For this review, take the finished solid that the model builds, in its own axes (mm). Face numbers are marked on the shaded views. A direction names the side the tool comes from. Round coordinates to 2 decimals unless told otherwise and drop trailing zeros. Loops run counter-clockwise (first coordinate to the right, second up) from the corner with the lowest first, then second, coordinate; pieces in that order, holes last. Notation, with made-up numbers: (51.25, -16.75) -> (100.25, -16.75) arc R26 ccw to (100.25, 18.25) -> close; hole circle Ø11 at (33, 31.5). An arc over 180 degrees is marked (long way). Write each question's results on one line, items separated by ' | '.
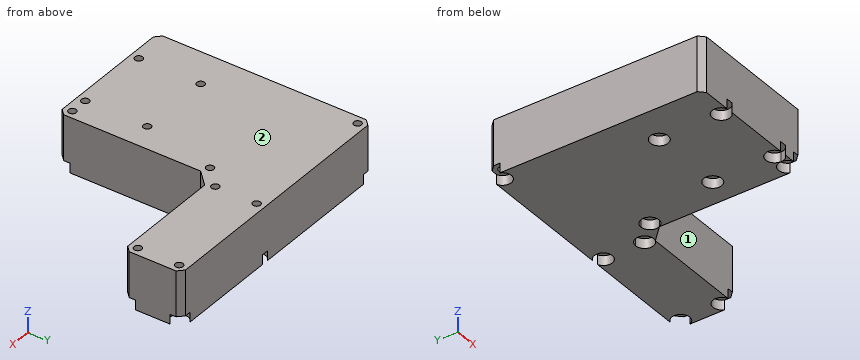
Autodesk Inventor part; units mm, degrees
ref_plane "Arbeitsebene2" through (-65, -116.035, 20) normal (0, 0, -1) x (0, 1, 0)
ref_plane "YZ Plane" through (0, 0, 0) normal (1, 0, 0) x (0, 1, 0)
ref_plane "XZ Plane" through (0, 0, 0) normal (0, 1, 0) x (-1, 0, 0)
ref_plane "Arbeitsebene1" through (0, 0, 0) normal (0, 0, 1) x (1, 0, 0)
ref_plane "Arbeitsebene2" through (-65, -116.035, 20) normal (0, 0, -1) x (0, 1, 0)
sketch "Skizze1" plane through (0, 0, 0) normal (0, 0, 1) x (1, 0, 0)
  circle A0 centre (-21, -24.715) radius 10
  circle A1 centre (-34.5, -13.465) radius 2
  circle A2 centre (-7.5, -13.465) radius 2
  circle A3 centre (-7.5, -35.965) radius 2
  circle A4 centre (-34.5, -35.965) radius 2
  circle A5 centre (-45, 35.965) radius 2
  circle A6 centre (-1, -35.965) radius 2
  circle A7 centre (-1, 14.0361) radius 2
  circle A8 centre (45, 35.965) radius 2
  circle A9 centre (45, 20.965) radius 2
  circle A10 centre (5.9289, 20.965) radius 2
  circle A11 centre (5.9289, 35.965) radius 2
  line L0 (2, -38.965) -> (-48, -38.965)
  line L1 (-48, -38.965) -> (-48, 38.965)
  line L2 (-48, 38.965) -> (48, 38.965)
  line L3 (48, 38.965) -> (48, 17.965)
  line L4 (48, 17.965) -> (7.1716, 17.965)
  line L5 (7.1716, 17.965) -> (2, 12.7934)
  line L6 (2, 12.7934) -> (2, -38.965)
  point P0 (0, 0)
extrude "Extrusion1" add sketch "Skizze1" along normal up to surface (20 mm away) contours A0 | A1 | A2 | A3 | A4 | A5 | A6 | A7 | A8 | A9 | A10 | A11 | L0 L1 L2 L3 L4 L5 L6
chamfer "Fasen1" distance 2 angle 45 5 edges at (-48, 38.965, 10) (-48, -38.965, 10) (48, 38.965, 10) (48, 17.965, 10) (2, -38.965, 10)
sketch "Skizze2" plane through (0, 0, 0) normal (0, 0, -1) x (-1, 0, 0)
  circle A0 centre (21, -24.715) radius 10
  circle A1 centre (34.5, -13.465) radius 2
  circle A2 centre (7.5, -13.465) radius 2
  circle A3 centre (7.5, -35.965) radius 2
  circle A4 centre (34.5, -35.965) radius 2
  circle A5 centre (45, 35.965) radius 2
  circle A6 centre (1, -35.965) radius 2
  circle A7 centre (1, 14.0361) radius 2
  circle A8 centre (-45, 35.965) radius 2
  circle A9 centre (-45, 20.965) radius 2
  circle A10 centre (-5.9289, 20.965) radius 2
  circle A11 centre (-5.9289, 35.965) radius 2
  line L0 (-2, -38.965) -> (48, -38.965)
  line L1 (48, -38.965) -> (48, 38.965)
  line L2 (48, 38.965) -> (-48, 38.965)
  line L3 (-48, 38.965) -> (-48, 17.965)
  line L4 (-48, 17.965) -> (-7.1716, 17.965)
  line L5 (-7.1716, 17.965) -> (-2, 12.7934)
  line L6 (-2, 12.7934) -> (-2, -38.965)
  point P0 (0, 0)
hole "Bohrung1" at (45, 35.965, 0) at (5.9289, 35.965, 0) at (5.9289, 20.965, 0) at (-1, 14.0361, 0) at (45, 20.965, 0) at (-45, 35.965, 0) at (-7.5, -13.465, 0) at (-34.5, -13.465, 0) at (-34.5, -35.965, 0) at (-7.5, -35.965, 0) at (-1, -35.965, 0) direction (0, 0, 1) diameter 2.8 depth 20 counterbore diameter 6.5 counterbore depth 3.5
properties part number "MIAB_Spacer"
1. Tool access review of the marked faces 1 and 2: name each direction out of +Z, -Z, +X, -X, +Y, -Y from which nothing blocks a thin tool from reaching the whole face with its end or side.
Values found:
face 1: +Z, -Z, +X, -Y | face 2: +Z, +X, -X, +Y, -Y
2. Consider section B-B (z = 11). Give the number of separate pieces and of enclosed holes in the cut face, plus the area to 3 significant figures.
Values found:
separate pieces: 1 | enclosed holes: 11 | area: 4,800 mm2
3. Consider section A-A (x = -34.5). State the section outline as (y, z) points (3 decimals), plus the area to 3 significant figures.
Values found:
outline: (-38.965, 3.5) -> (-37.365, 3.5) -> (-37.365, 20) -> (-38.965, 20) -> close; (-34.565, 3.5) -> (-32.715, 3.5) -> (-32.715, 0) -> (-16.715, 0) -> (-16.715, 3.5) -> (-14.865, 3.5) -> (-14.865, 20) -> (-34.565, 20) -> close; (-12.065, 3.5) -> (-10.215, 3.5) -> (-10.215, 0) -> (38.965, 0) -> (38.965, 20) -> (-12.065, 20) -> close | area: 1,420 mm2
4. To check wall thickness, follow probe 1 along X at (y, z) = (35, 8.5); probe 2 along Y at (x, z) = (-33.5, 9) (3 decimals); probe 3 along Z at (x, y) = (-34, -12). State the ranges of each line that lie inside material, in increasing order.
Values found:
probe 1: x = -48 to -46.01, -43.99 to 4.91, 6.94 to 43.99, 46.01 to 48 | probe 2: y = -38.965 to -36.945, -34.985 to -14.445, -12.485 to 38.965 | probe 3: z = 3.5 to 20
5. For pin 1 (3.5 mm diameter, centred on x = 5.93, y = 35.97, fed in from -Z); pin 2 (12 mm diameter, centred on y = 7.5, z = 5, fed in from +X); pin 3 (8 mm diameter, centred on y = -14, z = 6, fed in from +X), all flat-tipped, find the tip position at first contact; note any pin that passes through.
Values found:
pin 1: stops at z = 3.5 | pin 2: stops at x = 2.71 | pin 3: stops at x = 2
6. Consider section C-C (y = -25). State the section outline as (x, z) points.
Values found:
outline: (-48, 0) -> (2, 0) -> (2, 20) -> (-48, 20) -> close
7. Consider section D-D (x = 24.5). State the section outline as (y, z) points (3 decimals).
Values found:
outline: (17.965, 0) -> (38.965, 0) -> (38.965, 20) -> (17.965, 20) -> close
